CAD build for the part. Positions are in the model's coordinates, mm. Face numbers are marked on the shaded views. A direction names the side the tool comes from. Coordinates: 2 decimals unless noted, no trailing zeros. Order: outer loops, then holes, each group sorted by start corner. A loop starts at its lowest first (then second) coordinate and runs counter-clockwise, first axis right, second up.
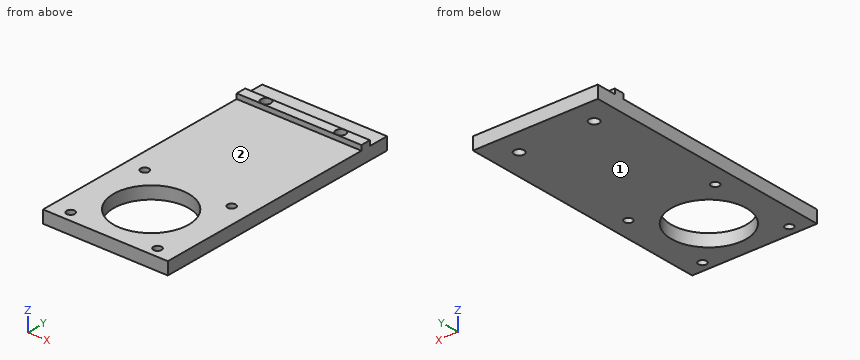
Autodesk Inventor part; units mm, degrees
ref_plane "YZ Plane" through (0, 0, 0) normal (1, 0, 0) x (0, 1, 0)
ref_plane "XZ Plane" through (0, 0, 0) normal (0, 1, 0) x (-1, 0, 0)
ref_plane "XY Plane" through (0, 0, 0) normal (0, 0, 1) x (1, 0, 0)
sketch "Sketch1" plane through (0, 0, 0) normal (0, 0, 1) x (1, 0, 0)
  line L0 (0, 144.2) -> (0, -144.2)
  line L1 (-70, 0) -> (70, 0)
  line L2 (-50, -103) -> (50, -103)
  line L3 (50, -103) -> (50, 103)
  line L4 (50, 103) -> (-50, 103)
  line L5 (-50, 103) -> (-50, -103)
  circle A0 centre (0, -60) radius 30
  circle A1 centre (-30, 83) radius 4
  circle A2 centre (30, 83) radius 4
  circle A3 centre (34.8, -94.8) radius 3.25
  circle A4 centre (34.8, -25.2) radius 3.25
  circle A5 centre (-34.8, -25.2) radius 3.25
  circle A6 centre (-34.8, -94.8) radius 3.25
  line L6 (-30, 83) -> (-30, 79)
  line L7 (0, -60) -> (0, -30)
  point P0 (0, 0)
  dimension "d2" = 60
  dimension "d4" = 8
  dimension "d0" = 100
  dimension "d1" = 206
  dimension "d3" = 43
  dimension "d5" = 8
  dimension "d6" = 20
  dimension "d7" = 20
  dimension "d8" = 20
  dimension "d9" = 20
  dimension "d10" = 6.5
  dimension "d11" = 6.5
  dimension "d12" = 6.5
  dimension "d13" = 6.5
  dimension "d14" = 69.6
  dimension "d15" = 69.6
  dimension "d16" = 69.6
  dimension "d17" = 69.6
  dimension "d18" = 0
  dimension "d19" = 0
  dimension "d20" = 34.8
  dimension "d21" = 34.8
  dimension "d22" = 109
extrude "Extrusion1" add sketch "Sketch1" along normal blind 20 contours A0 L0 L2 L5 L1 | L0 L1 L3 L2 A0 | L1 L5 L4 L0 | L0 L4 L3 L1
sketch "Sketch2" plane through (0, 0, 20) normal (0, 0, 1) x (1, 0, 0)
  line L0 (50, 103) -> (-50, 103)
  line L1 (-50, 103) -> (-50, -103)
  line L2 (-50, -103) -> (50, -103)
  line L3 (50, -103) -> (50, 103)
  circle A0 centre (30, 83) radius 4
  circle A1 centre (34.8, -25.2) radius 3.25
  circle A2 centre (34.8, -94.8) radius 3.25
  circle A3 centre (-34.8, -94.8) radius 3.25
  circle A4 centre (-34.8, -25.2) radius 3.25
  circle A5 centre (-30, 83) radius 4
  circle A6 centre (0, -60) radius 30
  line L4 (-50, 103) -> (-50, -103)
  line L5 (-50, 83) -> (50, 83)
  line L6 (-50, 87) -> (50, 87)
  line L7 (-50, 79) -> (50, 79)
  point P0 (0, 0)
  point P1 (50, 79)
  point P2 (-50, 79)
  point P3 (-50, 87)
  point P4 (50, 87)
  dimension "d25" = 4
  dimension "d26" = 4
extrude "Extrusion2" cut sketch "Sketch2" against normal blind 4 contours L3 L6 L1 L0 | L3 L2 L1 L7
sketch "Sketch3" plane through (0, 0, 0) normal (0, 0, -1) x (-1, 0, 0)
  line L0 (-50, 103) -> (50, 103)
  line L1 (-50, -103) -> (-50, 103)
  line L2 (50, -103) -> (-50, -103)
  line L3 (50, 103) -> (50, -103)
  circle A0 centre (-30, 83) radius 4
  circle A1 centre (-34.8, -25.2) radius 3.25
  circle A2 centre (-34.8, -94.8) radius 3.25
  circle A3 centre (34.8, -94.8) radius 3.25
  circle A4 centre (34.8, -25.2) radius 3.25
  circle A5 centre (30, 83) radius 4
  circle A6 centre (0, -60) radius 30
  point P0 (0, 0)
extrude "Extrusion3" cut sketch "Sketch3" against normal blind 6
properties part number "motor mount upper"
1) Slice it at B-B (z = 9.25). List the corners of the cut face in (x, y), plus the area to 3 significant figures.
2) Slice it at A-A (y = 83). List the corners of the cut face in (x, z).
3) Drill centre lines: probe 1 along Y at (x, z) = (34.8, 10.25); probe 2 along X at (y, z) = (-60, 10); probe 3 along Y at (x, z) = (0, 12.5). Where is each one in solid material? Low to high.
4) Which spindle directions (+Z, -Z, +X, -X, +Y, -Y) get a long thin tool onto all of the face, cutting with end or side? Do the marked faces 1 and 2. Say none if no direction does.
5) Slice it at D-D (x = 15). List the corners of the cut face in (y, z), plus the area to 3 significant figures.
6) Slice it at C-C (y = -60). List the corners of the cut face in (x, z), plus the area to 3 significant figures.
7) Pin check, flat tips, straight feed: P1, Ø10, axis at x = 2.5, y = 47.5, coming from the +Z side; P2, Ø3, axis at x = 17.5, z = 18, coming from the +Y side; P3, Ø6, axis at x = -34.8, y = -25.2, coming from the -Z side; P4, Ø2, axis at x = -13, z = 18, coming from the -Y side. Stop position of each tip, or through.
Worked out:
1. outline: (-50, -103) - (50, -103) - (50, 103) - (-50, 103) - close; hole circle Ø6.5 at (-34.8, -94.8); hole circle Ø6.5 at (-34.8, -25.2); hole circle Ø8 at (-30, 83); hole circle Ø60 at (0, -60); hole circle Ø8 at (30, 83); hole circle Ø6.5 at (34.8, -94.8); hole circle Ø6.5 at (34.8, -25.2)
1. area: 17,500 mm2
2. outline: (-50, 6) - (-34, 6) - (-34, 20) - (-50, 20) - close; (-26, 6) - (26, 6) - (26, 20) - (-26, 20) - close; (34, 6) - (50, 6) - (50, 20) - (34, 20) - close
3. probe 1: y = -103 to -98.05, -91.55 to -28.45, -21.95 to 103
3. probe 2: x = -50 to -30, 30 to 50
3. probe 3: y = -103 to -90, -30 to 103
4. face 1: -Z, +X, -X, +Y, -Y
4. face 2: +Z, +X, -X, -Y
5. outline: (-103, 6) - (-85.98, 6) - (-85.98, 16) - (-103, 16) - close; (-34.02, 6) - (103, 6) - (103, 16) - (87, 16) - (87, 20) - (79, 20) - (79, 16) - (-34.02, 16) - close
5. area: 1,570 mm2
6. outline: (-50, 6) - (-30, 6) - (-30, 16) - (-50, 16) - close; (30, 6) - (50, 6) - (50, 16) - (30, 16) - close
6. area: 400 mm2
7. P1: stops at z = 16
7. P2: stops at y = 87
7. P3: passes through
7. P4: stops at y = 79
